```python
from build123d import *

# Parameters (mm, degrees)
SKETCH_2_R           = 6
CUT_EXTRUDE_1_DEPTH  = 49.989794856
SKETCH_3_R           = 2.25
CUT_EXTRUDE_2_DEPTH  = 49.989794856
SKETCH_4_OUTSIDE_W   = 55.856
SKETCH_4_OUTSIDE_H   = 55.856
SKETCH_4_OUTSIDE_W_2 = 30
SKETCH_4_OUTSIDE_H_2 = 50.828583192
CUT_EXTRUDE_3_DEPTH  = 10
FILLET_1_R           = 1


with BuildPart() as part:
    # 草图1 → 旋转1 (revolve)
    with BuildSketch(Plane.XY):
        Polygon((0, 0), (0, 20), (10, 20), (10, 11), (40, 11), (40, 0), align=None)
    revolve(axis=Axis((40, 0, 0), (-1, 0, 0)))

    # 草图2 → 切除-拉伸1 (cut, through all)
    with BuildSketch(Plane.ZY):
        with Locations(Location((0, 0, 0), (0, 0, 270))):
            Circle(SKETCH_2_R)
    extrude(amount=-CUT_EXTRUDE_1_DEPTH, mode=Mode.SUBTRACT)

    # 草图3 → 切除-拉伸2 (cut, through all)
    with BuildSketch(Plane.ZY):
        with Locations(Location((0, 16, 0), (0, 0, 270))):
            Circle(SKETCH_3_R)
        with Locations(Location((11.313708499, 11.313708499, 0), (0, 0, 270))):
            Circle(SKETCH_3_R)
        with Locations(Location((11.313708499, -11.313708499, 0), (0, 0, 270))):
            Circle(SKETCH_3_R)
        with Locations(Location((0, -16, 0), (0, 0, 270))):
            Circle(SKETCH_3_R)
        with Locations(Location((-11.313708499, -11.313708499, 0), (0, 0, 270))):
            Circle(SKETCH_3_R)
        with Locations(Location((-11.313708499, 11.313708499, 0), (0, 0, 270))):
            Circle(SKETCH_3_R)
    extrude(amount=-CUT_EXTRUDE_2_DEPTH, mode=Mode.SUBTRACT)

    # 草图4 outside → 切除-拉伸3 (cut)
    with BuildSketch(Plane.ZY):
        Rectangle(SKETCH_4_OUTSIDE_W, SKETCH_4_OUTSIDE_H)
        Rectangle(SKETCH_4_OUTSIDE_W_2, SKETCH_4_OUTSIDE_H_2, mode=Mode.SUBTRACT)
    extrude(amount=-CUT_EXTRUDE_3_DEPTH, mode=Mode.SUBTRACT)

    # 圆角1
    fillet_1_edges = [part.edges().sort_by_distance(p)[0] for p in [
        (40, 6, 0),
        (0, 6, 0),
        (0, -20, 0),
        (0, 20, 0),
        (40, -11, 0),
    ]]
    fillet(fillet_1_edges, radius=FILLET_1_R)


solid = part.part
```
Geometry: final body of the model. Coordinates: model frame, mm. A direction names the side the tool comes from. Round coordinates to 2 decimals unless told otherwise and drop trailing zeros. Order: outer loops, then holes, each group sorted by start corner. A loop starts at its lowest first (then second) coordinate and runs counter-clockwise, first axis right, second up. Notation, with made-up numbers: (59, 50.25) - (64, 50.25) arc R31 cw to (64, 87.25) - close; hole circle Ø7 at (55, 78.5). An arc over 180 degrees is marked (long way). Use CSV: the item, a comma, the result in double quotes. Start each with the question number.
Q1. Access query for faces 1 (the face through (24.7, -2.38, 10.74)), 2 (the face through (4.93, -12.35, -13.31)). Directions: +Z, -Z, +X, -X, +Y, -Y. A direction counts if a zero-diameter tool reaches every point of the face in a straight line with its end or side. Return the directions, or none.
Q2. Mould query, pull axis Z, two halves, no side actions, for faces 3 (the face through (4.93, -18.146, 0.676)), 4 (the face through (6, 20, 0)), 5 (the face through (4.93, 13.854, 0.676)), 6 (the face through (40, 2, -7)). Classes: +Z half, -Z half, draft (parallel to the pull), parting line (faces both ways), or undercut.
Q3. Material intervals for line 1 along Z through (x, y) = (29, 0); line 2 along Z through (x, y) = (6, 3.5); line 3 along X through (y, z) = (17, -8.5), sorted ascending. Write a range as from..to.
Q4. Section query D-D (x = 37). Return loops of the section in (y, z), and give its area (3 significant figures).
Q5. Section query C-C (x = 6). Return loops of the section in (y, z).
Q6. Section query A-A (y = 0). Return loops of the section in (x, z).
Q7. Section query B-B (z = 0). Return loops of the section in (x, y).
Q8. First-contact query: pin 1 (12 mm diameter, centred on x = 28, y = 5.5, fed in from -Z); pin 2 (5 mm diameter, centred on x = 19.5, y = 12.5, fed in from -Z); pin 3 (1 mm diameter, centred on x = 13, z = 2.5, fed in from +Y); pin 4 (6 mm diameter, centred on y = -11.31, z = -11.31, fed in from -X). Flat tips, straight axial feed; report the tip coordinate or a pass-through.
Result set:
1,face 1,"+X"
1,face 2,"+X, -X"
2,face 3,"undercut"
2,face 4,"parting line"
2,face 5,"undercut"
2,face 6,"draft"
3,line 1,"z = -11..-6, 6..11"
3,line 2,"z = -15..-4.87, 4.87..15"
3,line 3,"x = 0..10"
4,outline,"circle Ø22 at (0, 0); hole circle Ø12 at (0, 0)"
4,area,"267 mm2"
5,outline,"(-13.23, -15) - (13.23, -15) arc R20 ccw to (13.23, 15) - (-13.23, 15) arc R20 ccw to start; hole circle Ø4.5 at (-16, 0); hole circle Ø4.5 at (-11.31, -11.31); hole circle Ø4.5 at (-11.31, 11.31); hole circle Ø12 at (0, 0); hole circle Ø4.5 at (11.31, -11.31); hole circle Ø4.5 at (11.31, 11.31); hole circle Ø4.5 at (16, 0)"
6,outline,"(0, -15) - (10, -15) - (10, -11) - (39, -11) arc R1 ccw to (40, -10) - (40, -7) arc R1 ccw to (39, -6) - (1, -6) arc R1 ccw to (0, -7) - close; (0, 7) arc R1 ccw to (1, 6) - (39, 6) arc R1 ccw to (40, 7) - (40, 10) arc R1 ccw to (39, 11) - (10, 11) - (10, 15) - (0, 15) - close"
7,outline,"(0, -19) arc R1 ccw to (1, -20) - (10, -20) - (10, -18.25) - (0, -18.25) - close; (0, -13.75) - (10, -13.75) - (10, -11) - (39, -11) arc R1 ccw to (40, -10) - (40, -7) arc R1 ccw to (39, -6) - (1, -6) arc R1 ccw to (0, -7) - close; (0, 7) arc R1 ccw to (1, 6) - (39, 6) arc R1 ccw to (40, 7) - (40, 10) arc R1 ccw to (39, 11) - (10, 11) - (10, 13.75) - (0, 13.75) - close; (0, 18.25) - (10, 18.25) - (10, 20) - (1, 20) arc R1 ccw to (0, 19) - close"
8,pin 1,"stops at z = -11"
8,pin 2,"stops at z = -4.58"
8,pin 3,"stops at y = 10.82"
8,pin 4,"stops at x = 0"
